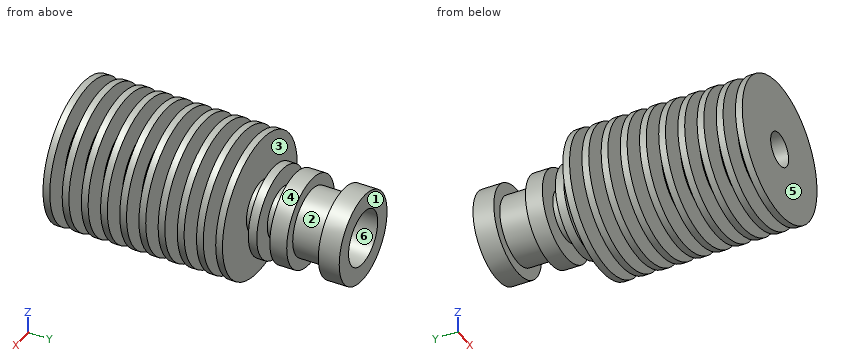
from build123d import *


with BuildPart() as part:
    # Sketch1 → Revolve1 (revolve)
    with BuildSketch(Plane.XY):
        Polygon((3, -25.05), (12.5, -25.05), (12.5, -23.85), (7.5, -23.85), (7.5, -21.65), (12.5, -21.65), (12.5, -20.45), (7.5, -20.45), (7.5, -18.25), (12.5, -18.25), (12.5, -17.05), (7.5, -17.05), (7.5, -14.85), (12.5, -14.85), (12.5, -13.65), (7.5, -13.65), (7.5, -11.45), (12.5, -11.45), (12.5, -10.25), (7.5, -10.25), (7.5, -8.05), (12.5, -8.05), (12.5, -6.85), (6.5, -6.85), (6.5, -4.65), (12.5, -4.65), (12.5, -3.45), (4.5, -3.45), (4.5, -1.25), (12.5, -1.25), (12.5, -0.05), (4.5, -0.05), (4.5, 2.15), (12.5, 2.15), (12.5, 3.35), (4.5, 3.35), (4.5, 5.55), (12.5, 5.55), (12.5, 6.75), (4.5, 6.75), (4.5, 8.95), (8, 8.95), (8, 10.45), (4.5, 10.45), (4.5, 12.75), (8, 12.75), (8, 15.75), (6, 15.75), (6, 21.35), (8, 21.35), (8, 25.05), (4.8641, 25.05), (4.8641, 15.05), (2, 10.089233282), (2, 6.089233282), (1, 5.511883013), (1, -5.895299462), (3, -7.05), align=None)
    revolve(axis=Axis((0, -25.05, 0), (0, 1, 0)))


solid = part.part
Work out the finished part from the listing and answer in its coordinate system (mm). Face numbers are marked on the shaded views. A direction names the side the tool comes from. Round coordinates to 2 decimals unless told otherwise and drop trailing zeros. Loops run counter-clockwise (first coordinate to the right, second up) from the corner with the lowest first, then second, coordinate; pieces in that order, holes last. Notation, with made-up numbers: (-2, 26) -> (38, 26) arc R25 cw to (38, 47) -> close; hole circle Ø10 at (16.5, 43.5). An arc over 180 degrees is marked (long way). Use one line per item in the form item = value.
(1) Find section B-B on z = -10.75. Give the number of separate pieces and of enclosed holes in the cut face, then the cut area to 3 significant figures.
Answer list:
separate_pieces = 10
enclosed_holes = 0
area = 153 mm2
(2) Flat-ended cylindrical pins translate along their axes: P1, Ø1.5, axis at y = 9.5, z = -7.5, coming from the +X side; P2, Ø12, axis at x = -6.5, y = -19, coming from the -Z side; P3, Ø2, axis at y = -1.5, z = -7, coming from the -X side. Find the tip coordinate at first contact, or state that the pin passes through.
Answer list:
P1 = 4.29
P2 = -12.49
P3 = -10.95
(3) For a pull along Y with two mould halves and no side action, classify the marked faces 1, 2, 3 and 4 as released by +Y, released by -Y, zero draft, split by the parting line, or undercut.
Answer list:
face_1 = released by +Y
face_2 = undercut
face_3 = undercut
face_4 = zero draft
(4) Straight lines are drawn through the part: line 1 (Z direction, x = 0, y = -14.25); line 2 (Z direction, x = 0, y = 19.5); line 3 (X direction, y = 22, z = 0). For each, find the intervals that lie inside material, in ascending order.
Answer list:
line_1 = -12.5 to -3, 3 to 12.5
line_2 = -6 to -4.86, 4.86 to 6
line_3 = -8 to -4.86, 4.86 to 8
(5) Find section D-D on y = -2.5. Give the vertices of the cut face in (x, z).
Answer list:
outline = circle Ø9 at (0, 0); hole circle Ø2 at (0, 0)
(6) A tool of negligible diameter and unlimited length cuts with its end or side. For the marked faces 5 and 6, from which of +Z, -Z, +X, -X, +Y, -Y can it reach the whole face along a straight path? Write none if from no direction.
Answer list:
face_5 = +Z, -Z, +X, -X, -Y
face_6 = +Y
(7) Find section A-A on y = -16. Give the vertices of the cut face in (x, z), then the cut area to 3 significant figures.
Answer list:
outline = circle Ø15 at (0, 0); hole circle Ø6 at (0, 0)
area = 148 mm2
